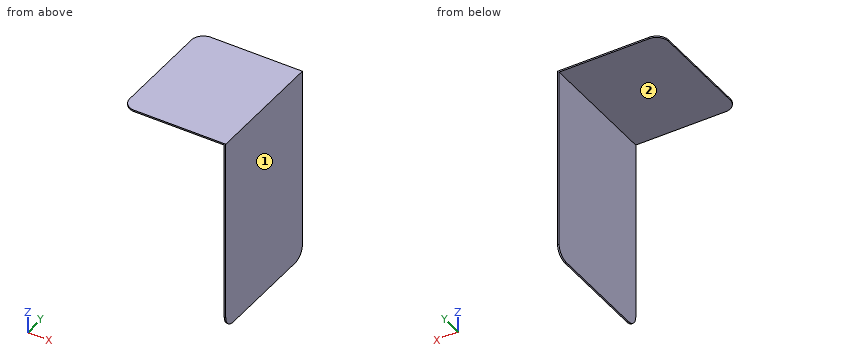
Autodesk Inventor part; units mm, degrees
ref_plane "YZ Plane" through (0, 0, 0) normal (1, 0, 0) x (0, 1, 0)
ref_plane "XZ Plane" through (0, 0, 0) normal (0, 1, 0) x (-1, 0, 0)
ref_plane "XY Plane" through (0, 0, 0) normal (0, 0, 1) x (1, 0, 0)
sketch "Sketch1" plane through (0, 0, 0) normal (0, 1, 0) x (-1, 0, 0)
  line L0 (0, 0) -> (0, -205.74)
  line L1 (0, 0) -> (109.22, 0)
  line L2 (1.5875, -205.74) -> (1.5875, -1.5875)
  line L3 (1.5875, -1.5875) -> (109.22, -1.5875)
  line L4 (109.22, 0) -> (109.22, -1.5875)
  line L5 (0, -205.74) -> (1.5875, -205.74)
  dimension "d0" = 205.74
  dimension "d1" = 109.22
  dimension "d2" = 1.5875
extrude "Extrusion1" add sketch "Sketch1" along normal blind 129.54
fillet "Fillet1" radius 12.7 4 edges at (-0.7938, 129.54, -205.74) (-0.7938, 0, -205.74) (-109.22, 129.54, -0.7937) (-109.22, 0, -0.7937)
properties part number "book_stand"
Part model, mm, in its own coordinate system. Face numbers are marked on the shaded views. A direction names the side the tool comes from. Give positions to 0.01 mm unless a question says otherwise; leave off trailing zeros. Write each loop counter-clockwise with the first axis right and the second up, starting at its lowest first coordinate (ties: lowest second). Pieces come first, ordered by that corner, then holes.
1) Probe L1, parallel to Z at x = -73, y = 57. List the from-to ranges inside material, lowest first.
Resolved:
L1: z = -1.59 to 0
2) Cut at A-A on y = 28. Write the cut outline in (x, z), then the cut area to 3 significant figures.
Resolved:
outline: (-109.22, -1.59) - (-1.59, -1.59) - (-1.59, -205.74) - (0, -205.74) - (0, 0) - (-109.22, 0) - close
area: 497 mm2
3) Which spindle directions (+Z, -Z, +X, -X, +Y, -Y) get a long thin tool onto all of the face, cutting with end or side? Do the marked faces 1 and 2. Say none if no direction does.
Resolved:
face 1: +Z, -Z, +X, +Y, -Y
face 2: -Z, -X, +Y, -Y
4) Cut at C-C on z = -138. Write the cut outline in (x, y), then the cut area to 3 significant figures.
Resolved:
outline: (-1.59, 0) - (0, 0) - (0, 129.54) - (-1.59, 129.54) - close
area: 206 mm2
5) Pin check, flat tips, straight feed: pin 1 (12 mm diameter, centred on x = -29.5, y = 41, fed in from -Z); pin 2 (8 mm diameter, centred on y = 76, z = -143, fed in from -X). Stop position of each tip, or through.
Resolved:
pin 1: stops at z = -1.59
pin 2: stops at x = -1.59
6) Cut at B-B on x = -45.5. Write the cut outline in (y, z), then the cut area to 3 significant figures.
Resolved:
outline: (0, -1.59) - (129.54, -1.59) - (129.54, 0) - (0, 0) - close
area: 206 mm2
